Geometry: final body of the model. Coordinates: model frame, mm. Face numbers are marked on the shaded views. Give positions to 0.01 mm unless a question says otherwise; leave off trailing zeros. Write each loop counter-clockwise with the first axis right and the second up, starting at its lowest first coordinate (ties: lowest second). Pieces come first, ordered by that corner, then holes.
from build123d import *

# Parameters (mm, degrees)
SKETCH_1_W        = 1990
SKETCH_1_H        = 300
EXTRUDE_371_DEPTH = 11.5
EXTRUDE_1_DEPTH   = 89
SKETCH_7_W        = 70
SKETCH_7_H        = 230
SKETCH_7_R        = 13
EXTRUDE_2_DEPTH   = 16


with BuildPart() as part:
    # 草图1 → Extrude 371 (new body)
    with BuildSketch(Plane.XY):
        with Locations((0, 150)):
            Rectangle(SKETCH_1_W, SKETCH_1_H)
    extrude(amount=EXTRUDE_371_DEPTH)

    # 草图2 → 凸台-拉伸1 (add)
    with BuildSketch(Plane.XY.offset(11.5)):
        Polygon((-995, 300), (995, 300), (995, 288.5), (940, 288.5), (940, 277.5), (860, 277.5), (860, 288.5), (-860, 288.5), (-860, 277.5), (-940, 277.5), (-940, 288.5), (-995, 288.5), align=None)
        Polygon((-995, 0), (995, 0), (995, 11.5), (940, 11.5), (940, 22.5), (860, 22.5), (860, 11.5), (-860, 11.5), (-860, 22.5), (-940, 22.5), (-940, 11.5), (-995, 11.5), align=None)
    extrude(amount=EXTRUDE_1_DEPTH)

    # 草图7 → 凸台-拉伸2 (add)
    # profile 1 of 2: a face of its own
    with BuildSketch(Plane(origin=(0, 0, 0), x_dir=(-1, 0, 0), z_dir=(0, 0, -1))):
        with Locations((300, 150)):
            Rectangle(SKETCH_7_W, SKETCH_7_H)
        with Locations((300, 230)):
            Circle(SKETCH_7_R, mode=Mode.SUBTRACT)
        with Locations((300, 150)):
            Circle(SKETCH_7_R, mode=Mode.SUBTRACT)
        with Locations((300, 70)):
            Circle(SKETCH_7_R, mode=Mode.SUBTRACT)
    # profile 2 of 2: a face of its own
    with BuildSketch(Plane(origin=(0, 0, 0), x_dir=(-1, 0, 0), z_dir=(0, 0, -1))):
        with Locations((-300, 150)):
            Rectangle(SKETCH_7_W, SKETCH_7_H)
        with Locations(Location((-300, 70, 0), (0, 0, 180))):
            Circle(SKETCH_7_R, mode=Mode.SUBTRACT)
        with Locations(Location((-300, 150, 0), (0, 0, 180))):
            Circle(SKETCH_7_R, mode=Mode.SUBTRACT)
        with Locations(Location((-300, 230, 0), (0, 0, 180))):
            Circle(SKETCH_7_R, mode=Mode.SUBTRACT)
    extrude(amount=EXTRUDE_2_DEPTH)


solid = part.part
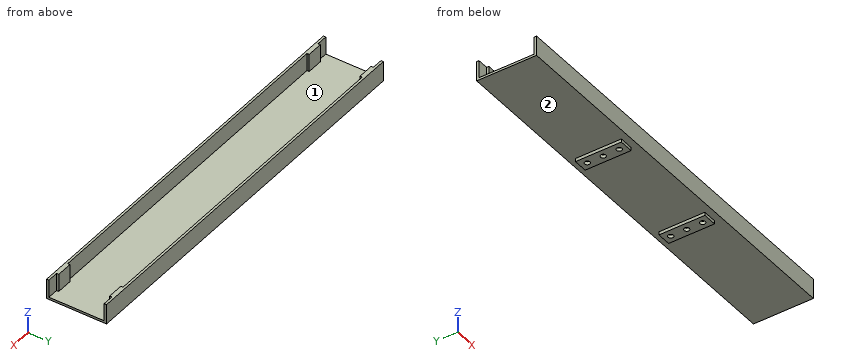
Q1. Ray query, line 1 along Y through (x, z) = (300, -11); line 2 along Y through (x, z) = (899.5, 77.5); line 3 along Y through (x, z) = (30.5, 44). Return the intervals inside material, ascending.
Filled sheet:
line 1: y = 35 to 57, 83 to 137, 163 to 217, 243 to 265
line 2: y = 0 to 22.5, 277.5 to 300
line 3: y = 0 to 11.5, 288.5 to 300
Q2. Pin query (flat end, axial travel): P1, Ø8, axis at x = -189, y = 257, coming from the -Z side; P2, Ø8, axis at y = 180.5, z = -6, coming from the -X side; P3, Ø13, axis at x = -302.5, z = -4.5, coming from the +Y side; P4, Ø4, axis at x = 185, y = 252.5, coming from the +Z side. Return the tip coordinate at first contact, or that it passes through.
Filled sheet:
P1: stops at z = 0
P2: stops at x = -335
P3: stops at y = 300
P4: stops at z = 11.5
Q3. Pull-direction query (Y, two-part tool) for the marked faces 1 and 2; classes: released by +Y, released by -Y, zero draft, split by the parting line, or undercut.
Filled sheet:
face 1: undercut
face 2: zero draft
Q4. Section A-A on z = 75. Output: boundary loops of the cut face in (x, y).
Filled sheet:
outline: (-995, 0) - (995, 0) - (995, 11.5) - (940, 11.5) - (940, 22.5) - (860, 22.5) - (860, 11.5) - (-860, 11.5) - (-860, 22.5) - (-940, 22.5) - (-940, 11.5) - (-995, 11.5) - close; (-995, 288.5) - (-940, 288.5) - (-940, 277.5) - (-860, 277.5) - (-860, 288.5) - (860, 288.5) - (860, 277.5) - (940, 277.5) - (940, 288.5) - (995, 288.5) - (995, 300) - (-995, 300) - close
Q5. Section B-B on x = 798. Output: boundary loops of the cut face in (y, z), plus the area to 3 significant figures.
Filled sheet:
outline: (0, 0) - (300, 0) - (300, 100.5) - (288.5, 100.5) - (288.5, 11.5) - (11.5, 11.5) - (11.5, 100.5) - (0, 100.5) - close
area: 5,500 mm2
